from build123d import *

# Parameters (mm, degrees)
SKETCH1_W             = 10
SKETCH1_H             = 40
BOSS_EXTRUDE1_DEPTH   = 2
M3X0_5_TAPPED_HOLE1_D = 2.5
CUT_EXTRUDE1_REACH    = 27.573
SKETCH6_R             = 1


with BuildPart() as part:
    # Sketch1 → Boss-Extrude1 (new body)
    with BuildSketch(Plane.XY):
        with Locations((0, -5)):
            Rectangle(SKETCH1_W, SKETCH1_H)
    extrude(amount=BOSS_EXTRUDE1_DEPTH)

    # M3x0.5 Tapped Hole1 (through all)
    with Locations(Plane.XY.offset(2)):
        with Locations((0, -0.164876805)):
            Hole(M3X0_5_TAPPED_HOLE1_D / 2)

    # Sketch6 → Cut-Extrude1 (cut, up to next)
    with BuildSketch(Plane.XY.offset(2), mode=Mode.PRIVATE) as cut_extrude1_sk1:
        with Locations((0, -23)):
            Circle(SKETCH6_R)
    cut_extrude1_tool1 = extrude(cut_extrude1_sk1.sketch, amount=-CUT_EXTRUDE1_REACH, mode=Mode.PRIVATE) & part.part
    add(cut_extrude1_tool1.solids().sort_by_distance((0, -23, 2))[0], mode=Mode.SUBTRACT)


solid = part.part
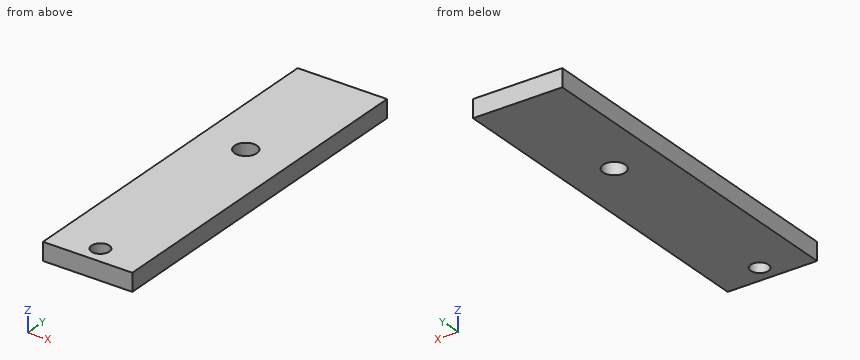
Input: part model. Units: mm. Frame: model coordinates. Give positions to 0.01 mm unless a question says otherwise; leave off trailing zeros. Loops run counter-clockwise (first coordinate to the right, second up) from the corner with the lowest first, then second, coordinate; pieces in that order, holes last. Notation, with made-up numbers: (-17, -19) -> (39, -19) arc R27 ccw to (39, 3) -> close; hole circle Ø2 at (40, 48.25). An arc over 180 degrees is marked (long way). Answer as a JSON object with one key per item and string values. Group by question number.
Item 1: Pin query (flat end, axial travel): P1, Ø1.6, axis at x = 0, y = -23, coming from the -Z side (3 decimals). Return the tip coordinate at first contact, or that it passes through.
Item 2: Cut plane D-D, the plane y = -1. Return the cut outline in (x, z), and give its area (3 significant figures).
Item 3: Cut plane B-B, the plane x = 0. Return the cut outline in (y, z).
Item 4: Line query: probe 1 along Y at (x, z) = (0, 1.5); probe 2 along X at (y, z) = (-1, 1.25). Output: solid intervals per line, ascending.
Item 5: Cut plane C-C, the plane z = 0.8. Return the cut outline in (x, y).
Item 6: Cut plane A-A, the plane y = -23. Return the cut outline in (x, z).
Checks:
{
 "1": {"P1": "passes through"},
 "2": {"outline": "(-5, 0) -> (-0.93, 0) -> (-0.93, 2) -> (-5, 2) -> close; (0.93, 0) -> (5, 0) -> (5, 2) -> (0.93, 2) -> close", "area": "16.3 mm²"},
 "3": {"outline": "(-25, 0) -> (-24, 0) -> (-24, 2) -> (-25, 2) -> close; (-22, 0) -> (-1.41, 0) -> (-1.41, 2) -> (-22, 2) -> close; (1.09, 0) -> (15, 0) -> (15, 2) -> (1.09, 2) -> close"},
 "4": {"probe 1": "y = -25 to -24, -22 to -1.41, 1.09 to 15", "probe 2": "x = -5 to -0.93, 0.93 to 5"},
 "5": {"outline": "(-5, -25) -> (5, -25) -> (5, 15) -> (-5, 15) -> close; hole circle Ø2.5 at (0, -0.16); hole circle Ø2 at (0, -23)"},
 "6": {"outline": "(-5, 0) -> (-1, 0) -> (-1, 2) -> (-5, 2) -> close; (1, 0) -> (5, 0) -> (5, 2) -> (1, 2) -> close"}
}
